from build123d import *

# Parameters (mm, degrees)
ESTRUSIONE_ESTRUSIONE1_DEPTH  = 100
TAGLIO_ESTRUSIONE5_DEPTH      = 518.911277836
TAGLIO_ESTRUSIONE5_DEPTH_BACK = 518.911277836
SCHIZZO2_R                    = 15
TAGLIO_ESTRUSIONE6_DEPTH      = 518.911277836
TAGLIO_ESTRUSIONE6_DEPTH_BACK = 518.911277836
SCHIZZO3_W                    = 85
SCHIZZO3_H                    = 100


with BuildPart() as part:
    # Schizzo1 → Estrusione-Estrusione1 (new body)
    with BuildSketch(Plane(origin=(0, 0, 0), x_dir=(1, 0, 0), z_dir=(0, 1, 0))):
        Polygon((-332.846822006, -200), (-332.846822006, 200), (467.153177994, 200), (467.153177994, 120), (-232.846822006, 120), (-232.846822006, -120), (467.153177994, -120), (467.153177994, -200), align=None)
    extrude(amount=ESTRUSIONE_ESTRUSIONE1_DEPTH)

    # Schizzo2 → Taglio-Estrusione5 (cut, two sides: drawn at the far end of the back side and taken through both)
    with BuildSketch(Plane.XY.offset(-TAGLIO_ESTRUSIONE5_DEPTH_BACK)):
        with Locations((-315.846822006, 50)):
            Circle(SCHIZZO2_R)
        with Locations((-150.146822006, 50)):
            Circle(SCHIZZO2_R)
        with Locations((449.853177994, 50)):
            Circle(SCHIZZO2_R)
    extrude(amount=TAGLIO_ESTRUSIONE5_DEPTH + TAGLIO_ESTRUSIONE5_DEPTH_BACK, mode=Mode.SUBTRACT)

    # Schizzo3 → Taglio-Estrusione6 (cut, two sides: drawn at the far end of the back side and taken through both)
    with BuildSketch(Plane(origin=(0, 0, 0), x_dir=(1, 0, 0), z_dir=(0, 1, 0)).offset(-TAGLIO_ESTRUSIONE6_DEPTH_BACK)):
        with Locations((-290.346822006, 0)):
            Rectangle(SCHIZZO3_W, SCHIZZO3_H)
    extrude(amount=TAGLIO_ESTRUSIONE6_DEPTH + TAGLIO_ESTRUSIONE6_DEPTH_BACK, mode=Mode.SUBTRACT)


solid = part.part
Design review of the part built by this model. Coordinates are the model's own, in mm. A direction names the side the tool comes from. Round coordinates to 2 decimals unless told otherwise and drop trailing zeros. Write each loop counter-clockwise with the first axis right and the second up, starting at its lowest first coordinate (ties: lowest second). Pieces come first, ordered by that corner, then holes.
Item 1: Consider section B-B on z = -150. Give the boundary of the cut face in (x, y), and give its area (3 significant figures).
Item 2: Consider section C-C on z = -85. Give the boundary of the cut face in (x, y).
Item 3: Consider section D-D on y = 16. Give the boundary of the cut face in (x, z).
Item 4: For pin 1 Ø1.5 at (x, z) = (239, -155.5) entering from -Y, flat-tipped, find the tip position at first contact; note if it passes through.
Item 5: Wall thickness on L1, parallel to X at y = 50, z = 159; L2, parallel to Z at x = -181.5, y = 54; L3, parallel to X at y = 57.5, z = -133: over which ranges is each line inside the solid? List them lowest first.
Item 6: Draft analysis for pull direction Z (two halves, no side actions). For faces 1 (the flat face through (112, 49, 120)), 2 (the flat face through (73, 0, -136)), 3 (the flat face through (73, 49, 200)), state which applies: released by +Z, released by -Z, zero draft, split by the parting line, or undercut.
Item 7: Consider section A-A on x = -267.5. Give the boundary of the cut face in (y, z).
Item 8: For faces 4 (the flat face through (122, 49, -120)), 5 (the cylindrical face through (438.8, 60.14, 159.44)), 6 (the flat face through (-291, 49, -50)), list the 3-axis set-ups (+Z, -Z, +X, -X, +Y, -Y) from which the entire face can be reached by the end or side of a thin tool; tool diameter is ignored.
Check values:
1. outline: (-332.85, 0) - (467.15, 0) - (467.15, 100) - (-332.85, 100) - close; hole circle Ø30 at (-315.85, 50); hole circle Ø30 at (-150.15, 50); hole circle Ø30 at (449.85, 50)
1. area: 77,900 mm2
2. outline: (-332.85, 0) - (-232.85, 0) - (-232.85, 100) - (-332.85, 100) - close; hole circle Ø30 at (-315.85, 50)
3. outline: (-332.85, -200) - (467.15, -200) - (467.15, -120) - (-232.85, -120) - (-232.85, 120) - (467.15, 120) - (467.15, 200) - (-332.85, 200) - (-332.85, 50) - (-247.85, 50) - (-247.85, -50) - (-332.85, -50) - close
4. pin 1: stops at y = 0
5. L1: x = -332.85 to -330.85, -300.85 to -165.15, -135.15 to 434.85, 464.85 to 467.15
5. L2: z = -200 to -120, 120 to 200
5. L3: x = -332.85 to -328.84, -302.86 to -163.14, -137.16 to 436.86, 462.84 to 467.15
6. face 1: undercut
6. face 2: zero draft
6. face 3: released by +Z
7. outline: (0, -200) - (100, -200) - (100, -50) - (0, -50) - close; (0, 50) - (100, 50) - (100, 200) - (0, 200) - close
8. face 4: +X, +Y, -Y
8. face 5: +Z, -Z
8. face 6: -X, +Y, -Y
